Source: three-view drawing plus pictorial views. Frame: mm from the lowest corner of the part. A direction names the side the tool comes from. Give positions to 0.01 mm unless a question says otherwise; leave off trailing zeros. Order: outer loops, then holes, each group sorted by start corner. A loop starts at its lowest first (then second) coordinate and runs counter-clockwise, first axis right, second up. Notation, with made-up numbers: (-20, -36) - (27, -36) arc R20 ccw to (27, -29) - close; hole circle Ø5 at (-27.75, -23). An arc over 180 degrees is marked (long way). Use CSV: the item, a comma, the result in double quotes.
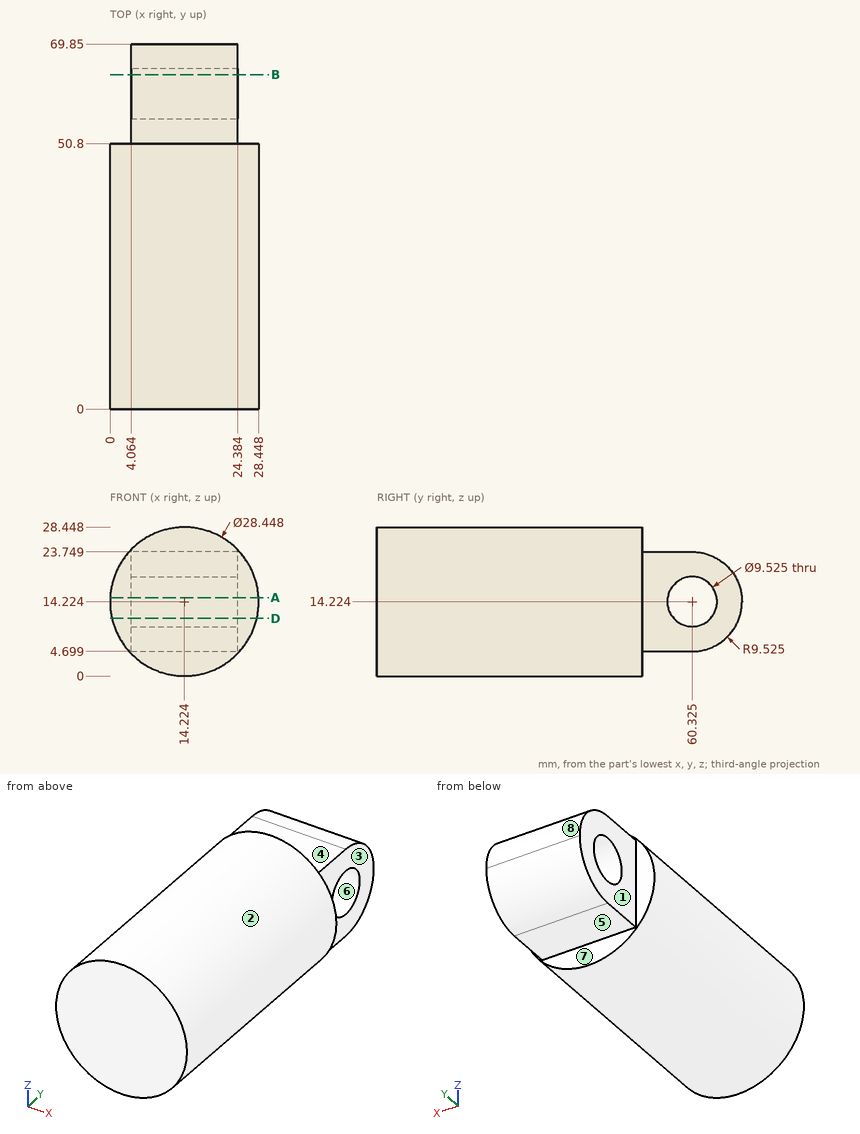
Item 1: Section A-A on z = 15. Return the cut outline in (x, y).
Filled in:
outline,"(0.02, 0) - (28.43, 0) - (28.43, 50.8) - (24.38, 50.8) - (24.38, 55.63) - (4.06, 55.63) - (4.06, 50.8) - (0.02, 50.8) - close; (4.06, 65.02) - (24.38, 65.02) - (24.38, 69.82) - (4.06, 69.82) - close"
Item 2: Material intervals for line 1 (Z direction, x = 20.5, y = 60.5); line 2 (Z direction, x = 7.75, y = 55.5); line 3 (X direction, y = 61.5, z = 23), sorted ascending. Write a range as from..to.
Filled in:
line 1,"z = 4.7..9.46, 18.98..23.75"
line 2,"z = 4.7..23.75"
line 3,"x = 4.06..24.38"
Item 3: Section D-D on z = 11. Return the cut outline in (x, y).
Filled in:
outline,"(0.37, 0) - (28.08, 0) - (28.08, 50.8) - (24.38, 50.8) - (24.38, 56.82) - (4.06, 56.82) - (4.06, 50.8) - (0.37, 50.8) - close; (4.06, 63.83) - (24.38, 63.83) - (24.38, 69.29) - (4.06, 69.29) - close"
Item 4: First-contact query: pin 1 (8 mm diameter, centred on y = 17.5, z = 4, fed in from +X); pin 2 (5 mm diameter, centred on x = 13, y = 58, fed in from -Z); pin 3 (5.5 mm diameter, centred on y = 61.5, z = 14, fed in from +X); pin 4 (6 mm diameter, centred on x = 20, y = 50.5, fed in from -Z). Flat tips, straight axial feed; report the tip coordinate or a pass-through.
Filled in:
pin 1,"stops at x = 27.01"
pin 2,"stops at z = 4.7"
pin 3,"passes through"
pin 4,"stops at z = 0.27"
Item 5: Set-up query: the marked faces 1, 2, 3, 4 and 5. Return all of +Z, -Z, +X, -X, +Y, -Y with unobstructed straight access to the full face (end or side cutting, diameter ignored); none if empty.
Filled in:
face 1,"+Z, -Z, -X, +Y"
face 2,"+Y, -Y"
face 3,"+Z, -Z, +X, +Y"
face 4,"+Z, +X, -X, +Y"
face 5,"-Z, +X, -X, +Y"
Item 6: Section B-B on y = 64. Return the cut outline in (x, z).
Filled in:
outline,"(4.06, 5.44) - (24.38, 5.44) - (24.38, 11.19) - (4.06, 11.19) - close; (4.06, 17.25) - (24.38, 17.25) - (24.38, 23.01) - (4.06, 23.01) - close"
Item 7: Mould query, pull axis Z, two halves, no side actions, for the marked faces 6, 7 and 8. Classes: released by +Z, released by -Z, zero draft, split by the parting line, or undercut.
Filled in:
face 6,"undercut"
face 7,"zero draft"
face 8,"released by +Z"
